from build123d import *

# Parameters (mm, degrees)
SKETCH2_R           = 8
SKETCH2_R_2         = 5
EXTRUDE_THIN1_DEPTH = 10
CUT_EXTRUDE1_DEPTH  = 10
SKETCH4_W           = 10
SKETCH4_H           = 10
BOSS_EXTRUDE1_DEPTH = 2
SKETCH5_R           = 3
CUT_EXTRUDE2_DEPTH  = 2
SKETCH6_W           = 25
SKETCH6_H           = 2
BOSS_EXTRUDE2_DEPTH = 2
SKETCH7_R           = 0.8
CUT_EXTRUDE3_DEPTH  = 2


with BuildPart() as part:
    # Sketch2 → Extrude-Thin1 (new body)
    with BuildSketch(Plane(origin=(0, 0, 0), x_dir=(1, 0, 0), z_dir=(0, 1, 0))):
        Circle(SKETCH2_R)
        Circle(SKETCH2_R_2, mode=Mode.SUBTRACT)
    extrude(amount=EXTRUDE_THIN1_DEPTH)

    # Sketch3 → Cut-Extrude1 (cut)
    with BuildSketch(Plane(origin=(0, 10, 0), x_dir=(1, 0, 0), z_dir=(0, 1, 0))):
        with BuildLine():
            Line((-8, 0), (8, 0))
            ThreePointArc((8, 0), (0, -8), (-8, 0))
        make_face()
    extrude(amount=-CUT_EXTRUDE1_DEPTH, mode=Mode.SUBTRACT)

    # Sketch4 → Boss-Extrude1 (add)
    with BuildSketch(Plane.XY):
        with Locations((10, 5)):
            Rectangle(SKETCH4_W, SKETCH4_H)
        with Locations((-10, 5)):
            Rectangle(SKETCH4_W, SKETCH4_H)
    extrude(amount=BOSS_EXTRUDE1_DEPTH)

    # Sketch5 → Cut-Extrude2 (cut)
    with BuildSketch(Plane(origin=(0, 0, 0), x_dir=(-1, 0, 0), z_dir=(0, 0, -1))):
        with Locations((-11.674262076, 5.406814048)):
            Circle(SKETCH5_R)
        with Locations((11.885931395, 5.406814048)):
            Circle(SKETCH5_R)
    extrude(amount=-CUT_EXTRUDE2_DEPTH, mode=Mode.SUBTRACT)

    # Sketch6 → Boss-Extrude2 (add)
    with BuildSketch(Plane(origin=(0, 10, 0), x_dir=(1, 0, 0), z_dir=(0, 1, 0))):
        with Locations((20.5, -1)):
            Rectangle(SKETCH6_W, SKETCH6_H)
    extrude(amount=BOSS_EXTRUDE2_DEPTH)

    # Sketch7 → Cut-Extrude3 (cut)
    with BuildSketch(Plane(origin=(0, 12, 0), x_dir=(1, 0, 0), z_dir=(0, 1, 0))):
        with Locations((16.5, -1.021213906)):
            Circle(SKETCH7_R)
    extrude(amount=-CUT_EXTRUDE3_DEPTH, mode=Mode.SUBTRACT)


solid = part.part
The model under review builds one solid part; all positions refer to its coordinate system, in mm. A direction names the side the tool comes from. Coordinates: 2 decimals unless noted, no trailing zeros. Loops run counter-clockwise (first coordinate to the right, second up) from the corner with the lowest first, then second, coordinate; pieces in that order, holes last. Notation, with made-up numbers: M 78.25,57.25 L 119.25,57.25 A12 cw 119.25,74.25 Z; hole C -35.5,0.25 d5. An arc over 180 degrees is marked long. Put each result on its own line as item: value. Start each with the question number.
Q1. The part is to be moulded in two halves that separate along X. For faces 1 (the flat face through (-5, 5, 1)), 2 (the flat face through (-2, 0, -5)), 3 (the flat face through (33, 11, 1)), 4 (the cylindrical face through (0, 5, -8)), say which applies: +X half, -X half, draft (parallel to the pull), parting line (faces both ways), or undercut.
Q2. Clearance check with flat-ended pins moving along their axes: pin 1 (1.5 mm diameter, centred on y = 8.5, z = 0.5, fed in from +X); pin 2 (5 mm diameter, centred on y = 4.5, z = -4, fed in from +X); pin 3 (3 mm diameter, centred on x = 10, y = 3, fed in from +Z); pin 4 (1.3 mm diameter, centred on x = 16.5, z = 1.02, fed in from -Y). State where each tip first meets the part, or that it passes through.
Q3. Add section C-C (z = -4). Write out the cut boundary in (x, y), and give its area (3 significant figures).
Q4. Add section B-B (y = 8). Write out the cut boundary in (x, z).
Q5. Add section D-D (y = 6). Write out the cut boundary in (x, z).
Q6. Wall thickness on line 1 (X direction, y = 9.25, z = -0.25); line 2 (Z direction, x = 0, y = 1.75); line 3 (Y direction, x = 5.5, z = 0.25): over which ranges is each line inside the solid? List them lowest first.
Q7. For faces 5 (the flat face through (15, 5, 1)), 6 (the flat face through (8, 11, 1)), 7 (the flat face through (14, 8, 0)), 8 (the flat face through (-9, 4, 0)), list the 3-axis set-ups (+Z, -Z, +X, -X, +Y, -Y) from which the entire face can be reached by the end or side of a thin tool; tool diameter is ignored.
Q8. Add section A-A (x = 16.5). Write out the cut boundary in (y, z).
Answers:
1. face 1: undercut
1. face 2: draft
1. face 3: +X half
1. face 4: parting line
2. pin 1: stops at x = 15
2. pin 2: stops at x = 7.86
2. pin 3: stops at z = 2
2. pin 4: passes through
3. outline: M -6.93,0 L -3,0 L -3,10 L -6.93,10 Z; M 3,0 L 6.93,0 L 6.93,10 L 3,10 Z
3. area: 78.6 mm^2
4. outline: M -15,0 L -13.39,0 L -13.39,2 L -15,2 Z; M -10.38,0 L -8,0 A8 ccw 8,0 L 10.17,0 L 10.17,2 L 5,2 L 5,0 A5 cw -5,0 L -5,2 L -10.38,2 Z; M 13.18,0 L 15,0 L 15,2 L 13.18,2 Z
5. outline: M -15,0 L -14.83,0 L -14.83,2 L -15,2 Z; M -8.95,0 L -8,0 A8 ccw 8,0 L 8.73,0 L 8.73,2 L 5,2 L 5,0 A5 cw -5,0 L -5,2 L -8.95,2 Z; M 14.62,0 L 15,0 L 15,2 L 14.62,2 Z
6. line 1: x = -8 to -4.99, 4.99 to 8
6. line 2: z = -8 to -5
6. line 3: y = 0 to 10
7. face 5: +Z, -Z, +X, -Y
7. face 6: +Z, -Z, -X, +Y
7. face 7: -Z, +X, +Y, -Y
7. face 8: -Z, -X, +Y, -Y
8. outline: M 10,0 L 12,0 L 12,0.22 L 10,0.22 Z; M 10,1.82 L 12,1.82 L 12,2 L 10,2 Z
